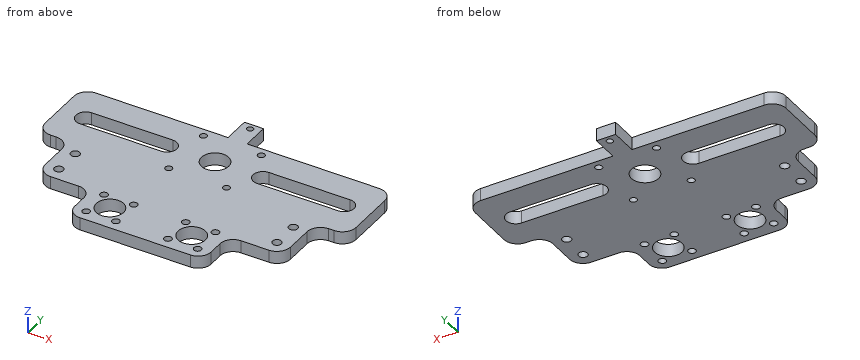
```python
from build123d import *

# Parameters (mm, degrees)
SKETCH1_W           = 144.78
SKETCH1_H           = 34.9885
BOSS_EXTRUDE1_DEPTH = 2.921
SKETCH2_R           = 6.35
SKETCH2_R_2         = 1.63195
CUT_EXTRUDE1_DEPTH  = 75.702676305
FILLET1_R           = 6.35
SKETCH3_W           = 114.3
SKETCH3_H           = 25.4
BOSS_EXTRUDE2_DEPTH = 5.842
FILLET2_R           = 6.35
SKETCH5_R           = 2.0828
CUT_EXTRUDE3_DEPTH  = 85.346652258
SKETCH6_W           = 8.89
SKETCH6_H           = 12.7
SKETCH6_R           = 1.4605
BOSS_EXTRUDE3_DEPTH = 5.842
SKETCH4_W           = 63.5
SKETCH4_H           = 19.05
BOSS_EXTRUDE4_DEPTH = 5.842
SKETCH7_R           = 6.35
CUT_EXTRUDE4_DEPTH  = 96.454340771
CIRPATTERN1_COUNT   = 4
FILLET3_R           = 6


with BuildPart() as part:
    # Sketch1 → Boss-Extrude1 (new, symmetric)
    with BuildSketch(Plane.XY):
        Rectangle(SKETCH1_W, SKETCH1_H)
        with BuildLine():
            Line((22.352, 4.572), (60.198, 4.572))
            ThreePointArc((60.198, 4.572), (64.77, 0), (60.198, -4.572))
            Line((60.198, -4.572), (22.352, -4.572))
            ThreePointArc((22.352, -4.572), (17.78, 0), (22.352, 4.572))
        make_face(mode=Mode.SUBTRACT)
        with BuildLine():
            Line((-22.352, 4.572), (-60.198, 4.572))
            ThreePointArc((-60.198, 4.572), (-64.77, 0), (-60.198, -4.572))
            Line((-60.198, -4.572), (-22.352, -4.572))
            ThreePointArc((-22.352, -4.572), (-17.78, 0), (-22.352, 4.572))
        make_face(mode=Mode.SUBTRACT)
    extrude(amount=BOSS_EXTRUDE1_DEPTH, both=True)

    # Sketch2 → Cut-Extrude1 (cut, through all)
    with BuildSketch(Plane.XY.offset(2.921)):
        Circle(SKETCH2_R)
        with Locations((13.470384182, -13.470384182)):
            Circle(SKETCH2_R_2)
        with Locations((-13.470384182, -13.470384182)):
            Circle(SKETCH2_R_2)
        with Locations((-13.470384182, 13.470384182)):
            Circle(SKETCH2_R_2)
        with Locations((13.470384182, 13.470384182)):
            Circle(SKETCH2_R_2)
    extrude(amount=-CUT_EXTRUDE1_DEPTH, mode=Mode.SUBTRACT)

    # Fillet1
    fillet1_edges = [part.edges().sort_by_distance(p)[0] for p in [
        (-72.39, 17.49425, 0),
        (72.39, 17.49425, 0),
        (72.39, -17.49425, 0),
        (-72.39, -17.49425, 0),
    ]]
    fillet(fillet1_edges, radius=FILLET1_R)

    # Sketch3 → Boss-Extrude2 (add)
    with BuildSketch(Plane.XY.offset(2.921)):
        with Locations((0, -30.19425)):
            Rectangle(SKETCH3_W, SKETCH3_H)
    extrude(amount=-BOSS_EXTRUDE2_DEPTH)

    # Fillet2
    fillet2_edges = [part.edges().sort_by_distance(p)[0] for p in [
        (-57.15, -42.89425, 0),
        (-57.15, -17.49425, 0),
        (57.15, -17.49425, 0),
        (57.15, -42.89425, 0),
    ]]
    fillet(fillet2_edges, radius=FILLET2_R)

    # Sketch5 → Cut-Extrude3 (cut, through all)
    with BuildSketch(Plane(origin=(0, 0, -2.921), x_dir=(-1, 0, 0), z_dir=(0, 0, -1))):
        with Locations((-50.8, -36.54425)):
            Circle(SKETCH5_R)
        with Locations((50.8, -36.54425)):
            Circle(SKETCH5_R)
        with Locations((50.8, -23.84425)):
            Circle(SKETCH5_R)
        with Locations((-50.8, -23.84425)):
            Circle(SKETCH5_R)
    extrude(amount=-CUT_EXTRUDE3_DEPTH, mode=Mode.SUBTRACT)

    # Sketch6 → Boss-Extrude3 (add)
    with BuildSketch(Plane(origin=(0, 0, -2.921), x_dir=(-1, 0, 0), z_dir=(0, 0, -1))):
        with Locations((0, 23.84425)):
            Rectangle(SKETCH6_W, SKETCH6_H)
        with Locations((0, 27.27325)):
            Circle(SKETCH6_R, mode=Mode.SUBTRACT)
    extrude(amount=-BOSS_EXTRUDE3_DEPTH)

    # Sketch4 → Boss-Extrude4 (add)
    with BuildSketch(Plane(origin=(0, 0, -2.921), x_dir=(-1, 0, 0), z_dir=(0, 0, -1))):
        with Locations((0, -52.41925)):
            Rectangle(SKETCH4_W, SKETCH4_H)
    extrude(amount=-BOSS_EXTRUDE4_DEPTH)

    # Sketch7 → Cut-Extrude4 (cut, through all)
    with BuildSketch(Plane(origin=(0, 0, -2.921), x_dir=(-1, 0, 0), z_dir=(0, 0, -1))):
        with Locations((-19.05, -49.809047213)):
            Circle(SKETCH7_R)
    cut_extrude4 = extrude(amount=-CUT_EXTRUDE4_DEPTH, mode=Mode.SUBTRACT)

    # Sketch9 → #6 Clearance Hole1 (revolve, cut)
    with BuildSketch(Plane(origin=(25.964797213, -42.89425, -2.921), x_dir=(0, 1, 0), z_dir=(1, 0, 0))):
        Polygon((0, 0), (0, 10.451068321), (1.7526, 9.398), (1.7526, 0), align=None)
    f_6_clearance_hole1 = revolve(axis=Axis((25.964797213, -42.89425, -9.271), (0, 0, 1)), mode=Mode.SUBTRACT)

    # CirPattern1: #6 Clearance Hole1 ×4 about axis
    cirpattern1_axis = Axis((19.05, -49.809047213, 0), (0, 0, 1))
    for i in range(1, CIRPATTERN1_COUNT):
        add(f_6_clearance_hole1.rotate(cirpattern1_axis, i * 360 / CIRPATTERN1_COUNT), mode=Mode.SUBTRACT)

    # Mirror1: Cut-Extrude4, #6 Clearance Hole1 across plane
    add(cut_extrude4.mirror(Plane.ZY), mode=Mode.SUBTRACT)
    add(f_6_clearance_hole1.mirror(Plane.ZY), mode=Mode.SUBTRACT)

    # Mirror1 copy 1 sketch → Mirror1 copy 1 (revolve, cut)
    with BuildSketch(Plane(origin=(-12.135202787, -42.89425, -2.921), x_dir=(1, 0, 0), z_dir=(0, 1, 0))):
        Polygon((0, 0), (0, -10.451068321), (1.7526, -9.398), (1.7526, 0), align=None)
    revolve(axis=Axis((-12.135202787, -42.89425, -9.271), (0, 0, -1)), mode=Mode.SUBTRACT)

    # Mirror1 copy 2 sketch → Mirror1 copy 2 (revolve, cut)
    with BuildSketch(Plane(origin=(-12.135202787, -56.723844426, -2.921), x_dir=(0, -1, 0), z_dir=(1, 0, 0))):
        Polygon((0, 0), (0, -10.451068321), (1.7526, -9.398), (1.7526, 0), align=None)
    revolve(axis=Axis((-12.135202787, -56.723844426, -9.271), (0, 0, -1)), mode=Mode.SUBTRACT)

    # Mirror1 copy 3 sketch → Mirror1 copy 3 (revolve, cut)
    with BuildSketch(Plane(origin=(-25.964797213, -56.723844426, -2.921), x_dir=(-1, 0, 0), z_dir=(0, -1, 0))):
        Polygon((0, 0), (0, -10.451068321), (1.7526, -9.398), (1.7526, 0), align=None)
    revolve(axis=Axis((-25.964797213, -56.723844426, -9.271), (0, 0, -1)), mode=Mode.SUBTRACT)

    # Fillet3
    fillet3_edges = [part.edges().sort_by_distance(p)[0] for p in [
        (31.75, -42.89425, 0),
        (31.75, -61.94425, 0),
        (-31.75, -61.94425, 0),
        (-31.75, -42.89425, 0),
    ]]
    fillet(fillet3_edges, radius=FILLET3_R)


solid = part.part
```
The listing builds one solid part. Answer for the finished solid, in the listing's coordinates (mm). Give positions to 0.01 mm unless a question says otherwise; leave off trailing zeros. Order: outer loops, then holes, each group sorted by start corner. A loop starts at its lowest first (then second) coordinate and runs counter-clockwise, first axis right, second up. Notation, with made-up numbers: (3.5, 87.5) -> (45.5, 87.5) arc R13 cw to (45.5, 98.5) -> close; hole circle Ø6 at (-38.5, 16). An arc over 180 degrees is marked (long way). Answer as a JSON object with one key per item and string values. Group by question number.
Item 1: The part is cut by section C-C on z = 1.45. Give the number of separate pieces and of enclosed holes in the cut face, and give its area (3 significant figures).
Item 2: Flat-ended cylindrical pins translate along their axes: pin 1 (1.8 mm diameter, centred on x = -28.5, z = -1, fed in from +Y); pin 2 (1.3 mm diameter, centred on x = 64.5, z = -1, fed in from -Y); pin 3 (3 mm diameter, centred on x = -40, z = 0, fed in from -Y). Find the tip coordinate at first contact, or state that the pin passes through.
Item 3: The part is cut by section A-A on y = 0. Write down the section's boundary in (x, z), and give its area (3 significant figures).
Item 4: The part is cut by section B-B on y = -53. Write down the section's boundary in (x, z), and give its area (3 significant figures).
Item 5: The part is cut by section D-D on y = 20.5. Write down the section's boundary in (x, z) (3 decimals).
Item 6: Consider L1, parallel to X at y = 0.5, z = 0.1; L2, parallel to Y at x = -50.8, z = 1; L3, parallel to X at y = -57, z = -1.7. Determine where each line is inside the solid, lowest interval first. Write a range as from..to.
Result set:
{
 "1": {"separate pieces": "1", "enclosed holes": "22", "area": "7,880 mm²"},
 "2": {"pin 1": "y = 17.49", "pin 2": "y = -17.49", "pin 3": "y = -42.89"},
 "3": {"outline": "(-72.39, -2.92) -> (-64.77, -2.92) -> (-64.77, 2.92) -> (-72.39, 2.92) -> close; (-17.78, -2.92) -> (-6.35, -2.92) -> (-6.35, 2.92) -> (-17.78, 2.92) -> close; (6.35, -2.92) -> (17.78, -2.92) -> (17.78, 2.92) -> (6.35, 2.92) -> close; (64.77, -2.92) -> (72.39, -2.92) -> (72.39, 2.92) -> (64.77, 2.92) -> close", "area": "223 mm²"},
 "4": {"outline": "(-31.75, -2.92) -> (-24.54, -2.92) -> (-24.54, 2.92) -> (-31.75, 2.92) -> close; (-13.56, -2.92) -> (13.56, -2.92) -> (13.56, 2.92) -> (-13.56, 2.92) -> close; (24.54, -2.92) -> (31.75, -2.92) -> (31.75, 2.92) -> (24.54, 2.92) -> close", "area": "243 mm²"},
 "5": {"outline": "(-4.445, -2.921) -> (4.445, -2.921) -> (4.445, 2.921) -> (-4.445, 2.921) -> close"},
 "6": {"L1": "-72.39..-64.74, -17.81..-6.33, 6.33..17.81, 64.74..72.39", "L2": "-42.89..-38.63, -34.46..-25.93, -21.76..-4.57, 4.57..17.49", "L3": "-31.66..-27.7, -24.23..-13.87, -10.4..10.4, 13.87..24.23, 27.7..31.66"}
}
